Source: CAD feature listing. Evaluate the final solid. Frame: model axes, mm. A direction names the side the tool comes from. Round coordinates to 2 decimals unless told otherwise and drop trailing zeros. Write each loop counter-clockwise with the first axis right and the second up, starting at its lowest first coordinate (ties: lowest second). Pieces come first, ordered by that corner, then holes. Notation, with made-up numbers: M -27.5,-25 L 4.5,-25 A22 cw 4.5,-1 Z; hole C -25,-36.5 d9. An arc over 180 degrees is marked long. Use a Markdown table: item, result.
```python
from build123d import *

# Parameters (mm, degrees)
SKETCH1_W           = 31
SKETCH1_H           = 29
BOSS_EXTRUDE1_DEPTH = 1.75
SKETCH2_R           = 2.25
BOSS_EXTRUDE2_DEPTH = 5.85
SKETCH3_W           = 31
SKETCH3_H           = 29
BOSS_EXTRUDE3_DEPTH = 1.75
SKETCH4_R           = 2.25
BOSS_EXTRUDE4_DEPTH = 4
SKETCH5_R           = 2.25
BOSS_EXTRUDE5_DEPTH = 4
SKETCH6_W           = 5.85
SKETCH6_H           = 2.3
BOSS_EXTRUDE6_DEPTH = 1.75


with BuildPart() as part:
    # Sketch1 → Boss-Extrude1 (new body)
    with BuildSketch(Plane(origin=(0, 0, 0), x_dir=(1, 0, 0), z_dir=(0, 1, 0))):
        Rectangle(SKETCH1_W, SKETCH1_H)
    extrude(amount=BOSS_EXTRUDE1_DEPTH)

    # Sketch2 → Boss-Extrude2 (add)
    with BuildSketch(Plane(origin=(0, 1.75, 0), x_dir=(1, 0, 0), z_dir=(0, 1, 0))):
        with Locations((-10, 10)):
            Circle(SKETCH2_R)
        with Locations((10, 10)):
            Circle(SKETCH2_R)
        with Locations((10, -10)):
            Circle(SKETCH2_R)
        with Locations((-10, -10)):
            Circle(SKETCH2_R)
    extrude(amount=BOSS_EXTRUDE2_DEPTH)

    # Sketch3 → Boss-Extrude3 (add)
    with BuildSketch(Plane(origin=(0, 7.6, 0), x_dir=(1, 0, 0), z_dir=(0, 1, 0))):
        Rectangle(SKETCH3_W, SKETCH3_H)
    extrude(amount=BOSS_EXTRUDE3_DEPTH)

    # Sketch4 → Boss-Extrude4 (add)
    with BuildSketch(Plane(origin=(0, 9.35, 0), x_dir=(1, 0, 0), z_dir=(0, 1, 0))):
        with Locations((-10, 10)):
            Circle(SKETCH4_R)
        with Locations((10, 10)):
            Circle(SKETCH4_R)
        with Locations((10, -10)):
            Circle(SKETCH4_R)
        with Locations((-10, -10)):
            Circle(SKETCH4_R)
    extrude(amount=BOSS_EXTRUDE4_DEPTH)

    # Sketch5 → Boss-Extrude5 (add)
    with BuildSketch(Plane.XZ):
        with Locations((10, 10)):
            Circle(SKETCH5_R)
        with Locations((10, -10)):
            Circle(SKETCH5_R)
        with Locations((-10, -10)):
            Circle(SKETCH5_R)
        with Locations((-10, 10)):
            Circle(SKETCH5_R)
    extrude(amount=BOSS_EXTRUDE5_DEPTH)

    # Sketch6 → Boss-Extrude6 (add)
    with BuildSketch(Plane.XZ):
        with Locations((3.425, 15.65)):
            Rectangle(SKETCH6_W, SKETCH6_H)
        with Locations((-3.425, 15.65)):
            Rectangle(SKETCH6_W, SKETCH6_H)
    extrude(amount=-BOSS_EXTRUDE6_DEPTH)


solid = part.part
```
Q1. First-contact query: pin 1 Ø0.9 at (y, z) = (1.5, 15) entering from +X; pin 2 Ø8.5 at (x, z) = (-3.5, -2) entering from +Y; pin 3 Ø0.9 at (y, z) = (1, 15.5) entering from -X; pin 4 Ø5 at (x, z) = (6.5, -7) entering from -Y. Flat tips, straight axial feed; report the tip coordinate or a pass-through.
Results are:
| item | result |
|---|---|
| pin 1 | x = 6.35 |
| pin 2 | y = 9.35 |
| pin 3 | x = -6.35 |
| pin 4 | y = -4 |
Q2. Section A-A on x = -1. Return loops of the section in (y, z), plus the area to 3 significant figures.
Results are:
| item | result |
|---|---|
| outline | M 0,-14.5 L 1.75,-14.5 L 1.75,16.8 L 0,16.8 Z; M 7.6,-14.5 L 9.35,-14.5 L 9.35,14.5 L 7.6,14.5 Z |
| area | 106 mm^2 |
Q3. Section B-B on z = -2. Return loops of the section in (x, y), plus the area to 4 significant figures.
Results are:
| item | result |
|---|---|
| outline | M -15.5,0 L 15.5,0 L 15.5,1.75 L -15.5,1.75 Z; M -15.5,7.6 L 15.5,7.6 L 15.5,9.35 L -15.5,9.35 Z |
| area | 108.5 mm^2 |
Q4. Line query: L1, parallel to Y at x = 5.5, z = 5.5; L2, parallel to Z at x = -9, y = 3.75; L3, parallel to X at y = -2.5, z = -8. Output: solid intervals per line, ascending.
Results are:
| item | result |
|---|---|
| L1 | 0 to 1.75, 7.6 to 9.35 |
| L2 | -12.02 to -7.98, 7.98 to 12.02 |
| L3 | -11.03 to -8.97, 8.97 to 11.03 |
Q5. Reachability of faces 4 (the cylindrical face through (8.34, 11.32, 8.48)), 5 (the flat face through (0, 1, 14.5)), 6 (the flat face through (-15.5, 1, 0)), 7 (the flat face through (-11, 1, 14.5)), 8 (the cylindrical face through (8.34, -1.97, -8.48)) from +Z, -Z, +X, -X, +Y, -Y: full face, straight path, thin tool, end or side. Return the list, or none.
Results are:
| item | result |
|---|---|
| face 4 | +Y |
| face 5 | +Z, +Y, -Y |
| face 6 | +Z, -Z, -X, +Y, -Y |
| face 7 | +Z, -X, +Y, -Y |
| face 8 | -Y |
Q6. Mould query, pull axis X, two halves, no side actions, for faces 1 (the flat face through (6.35, 1, 16)), 2 (the flat face through (-10, 13.35, -10)), 3 (the cylindrical face through (-11.66, 4.63, -11.52)). Classes: +X half, -X half, draft (parallel to the pull), parting line (faces both ways), or undercut.
Results are:
| item | result |
|---|---|
| face 1 | +X half |
| face 2 | draft |
| face 3 | undercut |
